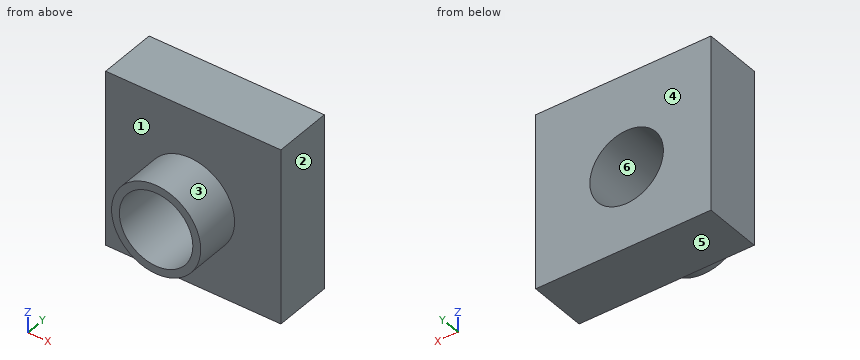
```python
from build123d import *

# Parameters (mm, degrees)
F0_W      = 101.6
F0_H      = 101.6
F0_R      = 25.850077
F1_DEPTH  = 25.4
F0_R_2    = 21.312016
F2_DEPTH  = 60.198
F1_FACE_W = 101.6
F1_FACE_H = 101.6
F1_FACE_R = 25.850077
F3_DEPTH  = 8.382


with BuildPart() as f1:
    # F0 (on Front) → F1 (new body)
    with BuildSketch(Plane.XZ):
        with Locations((1.916589, 3.479792)):
            Rectangle(F0_W, F0_H)
        Circle(F0_R, mode=Mode.SUBTRACT)
    extrude(amount=F1_DEPTH)

    # F0 (on Front) → F2 (join)
    with BuildSketch(Plane.XZ):
        Circle(F0_R)
        Circle(F0_R_2, mode=Mode.SUBTRACT)
    extrude(amount=F2_DEPTH)

    # F1_face (on face) → F3 (join)
    with BuildSketch(Plane(origin=(2.40587, -25.4, 4.368139), x_dir=(1, 0, 0), z_dir=(0, -1, 0))):
        with Locations((-0.489281, -0.888347)):
            Rectangle(F1_FACE_W, F1_FACE_H)
        with Locations((-2.40587, -4.368139)):
            Circle(F1_FACE_R, mode=Mode.SUBTRACT)
    extrude(amount=F3_DEPTH)


solid = f1.part
```
The model under review builds one solid part; all positions refer to its coordinate system, in mm. Face numbers are marked on the shaded views. A direction names the side the tool comes from. Give positions to 0.01 mm unless a question says otherwise; leave off trailing zeros. Write each loop counter-clockwise with the first axis right and the second up, starting at its lowest first coordinate (ties: lowest second). Pieces come first, ordered by that corner, then holes.
(1) The part is to be moulded in two halves that separate along Z. For the marked faces 3, 4, 5 and 6, say which applies: released by +Z, released by -Z, zero draft, split by the parting line, or undercut.
(2) Tool access review of the marked faces 1 and 2: name each direction out of +Z, -Z, +X, -X, +Y, -Y from which nothing blocks a thin tool from reaching the whole face with its end or side.
(3) Consider section A-A, the plane z = 0. Give the boundary of the cut face in (x, y), and give its area (3 significant figures).
(4) Consider section C-C, the plane y = -7.5. Give the boundary of the cut face in (x, z), and give its area (3 significant figures).
(5) Consider section B-B, the plane x = 0. Give the boundary of the cut face in (y, z), and give its area (3 significant figures).
(6) For P1, Ø4, axis at x = 38.5, z = -2, coming from the -Y side; P2, Ø1, axis at x = 22, y = -43, coming from the +Z side; P3, Ø3, axis at x = -2.5, y = -36.5, coming from the +Z side, all flat-tipped, find the tip position at first contact; note any pin that passes through.
(7) Consider section D-D, the plane x = -37.5. Give the boundary of the cut face in (y, z).
(8) To check wall thickness, follow L1, parallel to Z at x = 0, y = -15; L2, parallel to Y at x = -12.5, z = 50.5; L3, parallel to Z at x = 3.5, y = -17. State the ranges of each line that lie inside material, in increasing order.
Returned:
1. face 3: split by the parting line
1. face 4: zero draft
1. face 5: released by -Z
1. face 6: undercut
2. face 1: -Y
2. face 2: +Z, -Z, +X, +Y, -Y
3. outline: (-48.88, -33.78) - (-25.85, -33.78) - (-25.85, -60.2) - (-21.31, -60.2) - (-21.31, 0) - (-48.88, 0) - close; (21.31, -60.2) - (25.85, -60.2) - (25.85, -33.78) - (52.72, -33.78) - (52.72, 0) - (21.31, 0) - close
3. area: 2,230 mm2
4. outline: (-48.88, -47.32) - (52.72, -47.32) - (52.72, 54.28) - (-48.88, 54.28) - close; hole circle Ø42.62 at (0, 0)
4. area: 8,900 mm2
5. outline: (-60.2, -25.85) - (-33.78, -25.85) - (-33.78, -47.32) - (0, -47.32) - (0, -21.31) - (-60.2, -21.31) - close; (-60.2, 21.31) - (0, 21.31) - (0, 54.28) - (-33.78, 54.28) - (-33.78, 25.85) - (-60.2, 25.85) - close
5. area: 2,230 mm2
6. P1: stops at y = -33.78
6. P2: stops at z = 14.35
6. P3: stops at z = 25.83
7. outline: (-33.78, -47.32) - (0, -47.32) - (0, 54.28) - (-33.78, 54.28) - close
8. L1: z = -47.32 to -21.31, 21.31 to 54.28
8. L2: y = -33.78 to 0
8. L3: z = -47.32 to -21.02, 21.02 to 54.28
